```python
from build123d import *

# Parameters (mm, degrees)
F0_W         = 381
F0_H         = 381
F1_DEPTH     = 12.7
F3_W         = 144.018
F3_H         = 226.568
F4_DEPTH     = 38.1
F5_W         = 178.054
F5_H         = 87.376
F6_DEPTH     = 63.5
F7_W         = 127.762
F7_H         = 76.962
F8_DEPTH     = 25.146
F9_W         = 41.91
F9_H         = 68.1736
F10_DEPTH    = 26.035
F11_W        = 48.1622978261
F11_H        = 73.66
F12_DEPTH    = 38.1
F13_W        = 30.099
F13_H        = 69.85
F14_DEPTH    = 24.384
F15_T4_DEPTH = 466.4836595949
F15_T9_DEPTH = 466.4836595949
F16_W        = 71.074873209
F16_H        = 76.1698335409
F17_DEPTH    = 44.69176
F18_W        = 89.027
F18_H        = 87.376
F19_DEPTH    = 25.4
F20_W        = 32.1671016191
F20_H        = 87.376
F21_DEPTH    = 25.4
F22_W        = 48.1622978261
F22_H        = 29.0787754375
F22_H_2      = 26.581694724
F23_DEPTH    = 13.65146
F24_W        = 48.1622978261
F24_H        = 14.5393877187
F24_H_2      = 14.3073135987
F25_DEPTH    = 18.87303
F26_W        = 9.4362943637
F26_H        = 68.1736
F27_DEPTH    = 12.7
F28_R        = 2.54
F30_D        = 6.35
F31_R        = 5.08


# Not quite as in the source:
# - a fillet or chamfer that OpenCascade refuses, or shapes differently, is made with other operations: its cross-section is extruded or revolved along the edge and cut away or added


with BuildPart() as f1:
    # F0 (on Top) → F1 (new body)
    with BuildSketch(Plane.XY):
        Rectangle(F0_W, F0_H)
    extrude(amount=F1_DEPTH)

    # F3 (on face) → F4 (join)
    with BuildSketch(Plane.XY.offset(12.7)):
        with Locations((8.509, -26.416)):
            Rectangle(F3_W, F3_H)
    extrude(amount=F4_DEPTH)

    # F5 (on face) → F6 (join)
    with BuildSketch(Plane.XY.offset(12.7)):
        with Locations((75.1363011077, 134.6866802573)):
            Rectangle(F5_W, F5_H)
    extrude(amount=F6_DEPTH)

    # F7 (on face) → F8 (join)
    with BuildSketch(Plane.XY.offset(12.7)):
        with Locations((-101.4716736972, 140.4740017718)):
            Rectangle(F7_W, F7_H)
    extrude(amount=F8_DEPTH)

    # F9 (on face) → F10 (join)
    with BuildSketch(Plane.XY.offset(12.7)):
        with Locations((-139.3904201686, 51.5634464747)):
            Rectangle(F9_W, F9_H)
    extrude(amount=F10_DEPTH)

    # F11 (on face) → F12 (join)
    with BuildSketch(Plane.XY.offset(12.7)):
        with Locations((123.9150092006, 48.8317962736)):
            Rectangle(F11_W, F11_H)
    extrude(amount=F12_DEPTH)

    # F13 (on face) → F14 (join)
    with BuildSketch(Plane.XY.offset(12.7)):
        with Locations((-115.685201868, -34.925)):
            Rectangle(F13_W, F13_H)
        with Locations((-115.685201868, -116.3742716573)):
            Rectangle(F13_W, F13_H)
        with Locations((115.685201868, -34.925)):
            Rectangle(F13_W, F13_H)
        with Locations((115.685201868, -116.3742716573)):
            Rectangle(F13_W, F13_H)
    extrude(amount=F14_DEPTH)

    # F15: fillet of radius 49.2649730808 on 2 edges, made by hand


with BuildPart() as f15_tool2:
    # F15_s3 → F15_t4 (new body)
    with BuildSketch(Plane.XZ.offset(259.6578297975)):
        with BuildLine():
            ThreePointArc((80.518, 12.7), (63.1697785132, 40.1166266199), (32.534868081, 50.8))
            Line((32.534868081, 50.8), (80.518, 50.8))
            Line((80.518, 50.8), (80.518, 12.7))
        make_face()
    extrude(amount=-F15_T4_DEPTH)

    split(bisect_by=Plane.XZ.offset(-90.9986802573), keep=Keep.TOP)


with BuildPart() as f1_1:
    add(f1.part)

    # F15_t1: cut F15_tool2
    add(f15_tool2.part, mode=Mode.SUBTRACT)


with BuildPart() as f15_tool7:
    # F15_s8 → F15_t9 (new body)
    with BuildSketch(Plane.XZ.offset(-206.8258297975)):
        with BuildLine():
            ThreePointArc((-63.5, 12.7), (-46.1517785132, 40.1166266199), (-15.516868081, 50.8))
            Line((-15.516868081, 50.8), (-63.5, 50.8))
            Line((-63.5, 50.8), (-63.5, 12.7))
        make_face()
    extrude(amount=F15_T9_DEPTH)

    split(bisect_by=Plane.XZ.offset(-101.9930017718), keep=Keep.TOP)


with BuildPart() as f1_2:
    add(f1_1.part)

    # F15_t6: cut F15_tool7
    add(f15_tool7.part, mode=Mode.SUBTRACT)

    # F16 (on face) → F17 (cut)
    with BuildSketch(Plane.XY.offset(76.2)):
        with Locations((119.8119372129, 134.7657069564)):
            Rectangle(F16_W, F16_H)
    extrude(amount=-F17_DEPTH, mode=Mode.SUBTRACT)

    # F18 (on face) → F19 (cut)
    with BuildSketch(Plane.XY.offset(76.2)):
        with Locations((30.6228011077, 134.6866802573)):
            Rectangle(F18_W, F18_H)
    extrude(amount=-F19_DEPTH, mode=Mode.SUBTRACT)

    # F20 (on face) → F21 (cut)
    with BuildSketch(Plane.XY.offset(50.8)):
        with Locations((2.1928519172, 134.6866802573)):
            Rectangle(F20_W, F20_H)
    extrude(amount=-F21_DEPTH, mode=Mode.SUBTRACT)

    # F22 (on face) → F23 (cut)
    with BuildSketch(Plane.XY.offset(50.8)):
        with Locations((123.9150092006, 71.1224085549)):
            Rectangle(F22_W, F22_H)
        with Locations((123.9150092006, 25.2926436356)):
            Rectangle(F22_W, F22_H_2)
    extrude(amount=-F23_DEPTH, mode=Mode.SUBTRACT)

    # F24 (on face) → F25 (cut)
    with BuildSketch(Plane.XY.offset(37.14854)):
        with Locations((123.9150092006, 78.3921024142)):
            Rectangle(F24_W, F24_H)
        with Locations((123.9150092006, 18.045573961)):
            Rectangle(F24_W, F24_H_2)
    extrude(amount=-F25_DEPTH, mode=Mode.SUBTRACT)

    # F26 (on face) → F27 (cut)
    with BuildSketch(Plane.XY.offset(38.735)):
        with Locations((-155.6272729868, 51.5634464747)):
            Rectangle(F26_W, F26_H)
    extrude(amount=-F27_DEPTH, mode=Mode.SUBTRACT)

    # F28
    f28_edges = [f1_2.edges().sort_by_distance(p)[0] for p in [
        (-150.909126, 51.563446, 26.035),
        (-160.34542, 51.563446, 26.035),
        (-150.909126, 51.563446, 38.735),
        (-134.672273, 17.476646, 38.735),
        (-118.43542, 51.563446, 38.735),
        (-134.672273, 85.650246, 38.735),
        (-118.43542, 17.476646, 25.7175),
        (32.534868, -26.416, 50.8),
        (8.509, -139.7, 50.8),
        (-15.516868, -26.416, 50.8),
        (8.509, 86.868, 50.8),
        (-160.34542, 17.476646, 19.3675),
        (-160.34542, 85.650246, 19.3675),
        (-118.43542, 85.650246, 25.7175),
        (63.169779, 86.868, 40.116627),
        (63.169779, -139.7, 40.116627),
        (-46.151779, -139.7, 40.116627),
        (-46.151779, 86.868, 40.116627),
    ]]
    fillet(f28_edges, radius=F28_R)

    # F30 (through all)
    with Locations(Plane.XY.offset(12.7)):
        with Locations((-69.85, -177.6871830225), (69.85, -177.6871830225), (69.85, 184.4432204962), (-69.85, 184.4432204962)):
            Hole(F30_D / 2)

    # F31
    f31_edges = [f1_2.edges().sort_by_distance(p)[0] for p in [
        (-37.590674, 101.993002, 25.273),
        (-165.352674, 101.993002, 25.273),
        (-165.352674, 178.955002, 25.273),
        (-37.590674, 178.955002, 25.273),
    ]]
    fillet(f31_edges, radius=F31_R)


solid = f1_2.part
```
Here's how the part is built. I have some questions about the finished solid (model axes, mm). A direction names the side the tool comes from. Coordinates: 2 decimals unless noted, no trailing zeros. Loops run counter-clockwise (first coordinate to the right, second up) from the corner with the lowest first, then second, coordinate; pieces in that order, holes last. Notation, with made-up numbers: (67.25, 24) - (108.25, 24) arc R29 ccw to (108.25, 57) - close; hole circle Ø6 at (82.5, 3.5). An arc over 180 degrees is marked (long way). Return JSON: item names as keys, results as strings. Group by question number.
Item 1: Will these pins go through, and if not, where does the flat tip stop? P1, Ø12, axis at y = -44.5, z = 20.5, coming from the +X side; P2, Ø6, axis at y = -88, z = 22.5, coming from the -X side; P3, Ø2, axis at y = 15, z = 47.5, coming from the +X side.
Item 2: If we section it at D-D on y = 6: Write out the boundary of the cut face in (x, z).
Item 3: On a 3-axis mill with a long thin cutter (end or side, diameter ignored), from which of +Z, -Z, +X, -X, +Y, -Y can I reach the whole of each face in a straight line? I mean faces 1 (the face through (124, 56.583, 44)), 2 (the face through (-140, 17.477, 24)), 3 (the face through (-130.735, -117, 25)), 4 (the face through (2, 135, 25.4)). Say none if no direction works.
Item 4: I need wall thicknesses on line 1 (Y direction, x = -69.85, z = 6.25); line 2 (X direction, y = 133.5, z = 54.5); line 3 (X direction, y = 143, z = 45). Which ranges of each line are inside material? Lowest first, please. Write a range as from..to.
Item 5: If we section it at C-C on y = -62.5: Write out the boundary of the cut face in (x, z).
Item 6: We'd pull the mould along X, two halves only. Please class faces 5 (the face through (63.53, -27.97, 39.83)), 6 (the face through (-3, 3, 0)), 7 (the face through (-165.353, 140, 25)): +X half, -X half, draft (parallel to the pull), parting line (faces both ways), or undercut.
Item 7: If we section it at A-A on z = 55.5: Write out the boundary of the cut face in (x, y), and give its area (3 significant figures).
Calculated:
{
 "1": {"P1": "stops at x = 130.73", "P2": "stops at x = -130.73", "P3": "stops at x = 52.66"},
 "2": {"outline": "(-190.5, 0) - (190.5, 0) - (190.5, 12.7) - (80.52, 12.7) arc R49.26 ccw to (32.53, 50.8) - (-15.52, 50.8) arc R49.26 ccw to (-63.5, 12.7) - (-190.5, 12.7) - close"},
 "3": {"face 1": "+Z, +X", "face 2": "+Z, -X", "face 3": "+Z, -X, -Y", "face 4": "+Z, +Y"},
 "4": {"line 1": "y = -190.5..-180.86, -174.51..181.27, 187.62..190.5", "line 2": "x = 75.14..84.27, 155.35..164.16", "line 3": "x = 18.28..84.27, 155.35..164.16"},
 "5": {"outline": "(-190.5, 0) - (190.5, 0) - (190.5, 12.7) - (130.73, 12.7) - (130.73, 37.08) - (100.64, 37.08) - (100.64, 12.7) - (80.52, 12.7) arc R49.26 ccw to (32.53, 50.8) - (-15.52, 50.8) arc R49.26 ccw to (-63.5, 12.7) - (-100.64, 12.7) - (-100.64, 37.08) - (-130.73, 37.08) - (-130.73, 12.7) - (-190.5, 12.7) - close"},
 "6": {"face 5": "undercut", "face 6": "draft", "face 7": "-X half"},
 "7": {"outline": "(75.14, 91) - (164.16, 91) - (164.16, 178.37) - (75.14, 178.37) - close; hole (84.27, 96.68) - (155.35, 96.68) - (155.35, 172.85) - (84.27, 172.85) - close", "area": "2,370 mm^2"}
}
